The figure shows three views and two pictorial views of one solid part (mm, origin at its lowest corner). Answer the questions. A direction names the side the tool comes from. Give positions to 0.01 mm unless a question says otherwise; leave off trailing zeros. Loops run counter-clockwise (first coordinate to the right, second up) from the corner with the lowest first, then second, coordinate; pieces in that order, holes last. Notation, with made-up numbers: (1.5, 88) -> (16.5, 88) arc R17 ccw to (16.5, 116) -> close; hole circle Ø10 at (29.25, 41.5). An arc over 180 degrees is marked (long way). Answer as CSV lines item,"result". Start each with the question number.
1. Flat-ended cylindrical pins translate along their axes: pin 1 Ø2 at (x, y) = (88.5, 4) entering from -Z; pin 2 Ø12 at (x, z) = (22, 75) entering from +Y; pin 3 Ø10 at (x, z) = (110, 30) entering from -Y. Find the tip coordinate at first contact, or state that the pin passes through.
2. Find section B-B, the plane y = 3.75. Give the vertices of the cut face in (x, z).
3. Find the intervals of material crossed by line 1 along Y through (x, z) = (79, 16); line 2 along Y through (x, z) = (105, 17); line 3 along X through (y, z) = (4.5, 45.5), in increasing order.
4. Find section C-C, the plane x = 75.5. Give the vertices of the cut face in (y, z).
5. A tool of negligible diameter and unlimited length cuts with its end or side. For the marked faces 1, 2 and 3, from which of +Z, -Z, +X, -X, +Y, -Y can it reach the whole face along a straight path? Write none if from no direction.
6. Find section A-A, the plane z = 62.5. Give the vertices of the cut face in (x, y).
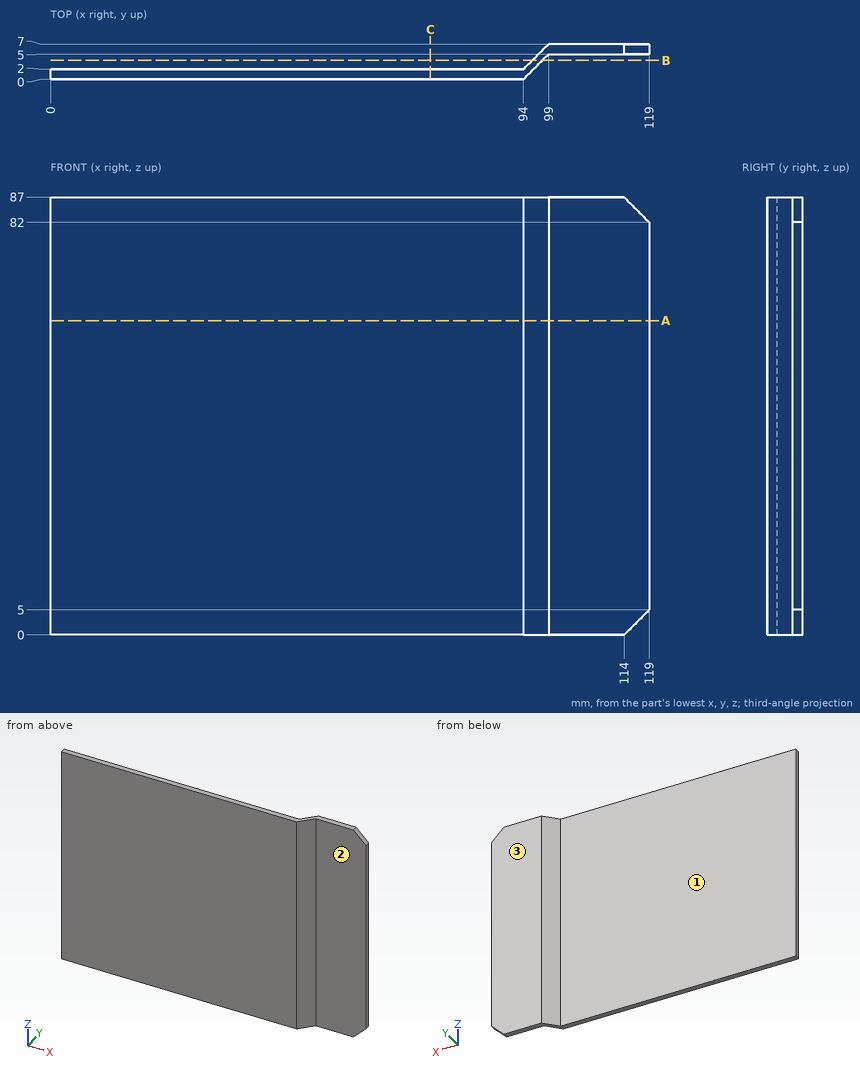
Resolved:
1,pin 1,"passes through"
1,pin 2,"stops at y = 2"
1,pin 3,"stops at y = 5"
2,outline,"(95.75, 0) -> (97.75, 0) -> (97.75, 87) -> (95.75, 87) -> close"
3,line 1,"y = 0 to 2"
3,line 2,"y = 5 to 7"
3,line 3,"x = 96.5 to 98.5"
4,outline,"(0, 0) -> (2, 0) -> (2, 87) -> (0, 87) -> close"
5,face 1,"+Z, -Z, -X, +Y"
5,face 2,"+Z, -Z, +X, -Y"
5,face 3,"+Z, -Z, +X, -X, +Y"
6,outline,"(0, 0) -> (94, 0) -> (99, 5) -> (119, 5) -> (119, 7) -> (99, 7) -> (94, 2) -> (0, 2) -> close"
